Source: CAD feature listing. Evaluate the final solid. Frame: model axes, mm. Coordinates: 2 decimals unless noted, no trailing zeros.
Item 1: Ray query, line 1 (Z direction, x = 0, y = -3); line 2 (X direction, y = -7.5, z = 247.65); line 3 (Z direction, x = -15, y = -7). Return the intervals inside material, ascending.
Item 2: Contact query for flat-ended pins moving along their axis: P1, Ø5.5, axis at x = 0, z = 247.65, coming from the -Y side; P2, Ø3, axis at x = 0.5, y = -6.5, coming from the +Z side. Output: stop coordinate, or through.
Item 3: Section A-A on y = -5. State how many separate pieces and enclosed holes the cut face has, then the cut area to 3 significant figures.
from build123d import *

# Parameters (mm, degrees)
F0_W     = 50.8
F0_H     = 19.05
F1_DEPTH = 927.1
F2_W     = 122.43557321
F2_H     = 50.8
F2_W_2   = 343.1604206562
F3_DEPTH = 25.4
F4_R     = 4.7625
F5_DEPTH = 25.4


# Not quite as in the source:
# - a feature names something its author has since deleted; it is built from what else it names


with BuildPart() as f1:
    # F0 (on Top) → F1 (new body)
    with BuildSketch(Plane.XY):
        Rectangle(F0_W, F0_H)
    extrude(amount=F1_DEPTH)

    # F2 (on Front) → F3 (cut)
    with BuildSketch(Plane.XZ):
        with Locations((22.4465244144, 177.8)):
            Rectangle(F2_W, F2_H)
        with Locations((-38.7818217278, 901.7)):
            Rectangle(F2_W_2, F2_H)
    extrude(amount=F3_DEPTH, mode=Mode.SUBTRACT)

    # F4 (on Front) → F5 (cut)
    with BuildSketch(Plane.XZ):
        with Locations((0, 247.65)):
            Circle(F4_R)
    extrude(amount=F5_DEPTH, mode=Mode.SUBTRACT)


solid = f1.part
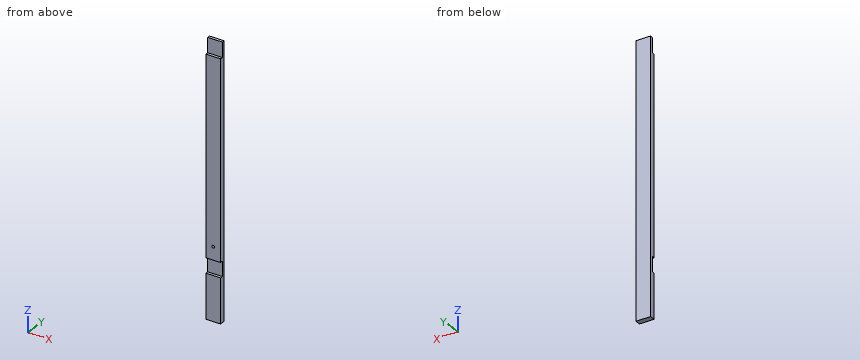
Answer list:
1. line 1: z = 0 to 152.4, 203.2 to 242.89, 252.41 to 876.3
1. line 2: x = -25.4 to -4.76, 4.76 to 25.4
1. line 3: z = 0 to 152.4, 203.2 to 876.3
2. P1: stops at y = 0
2. P2: stops at z = 876.3
3. separate pieces: 2
3. enclosed holes: 1
3. area: 41,900 mm2
